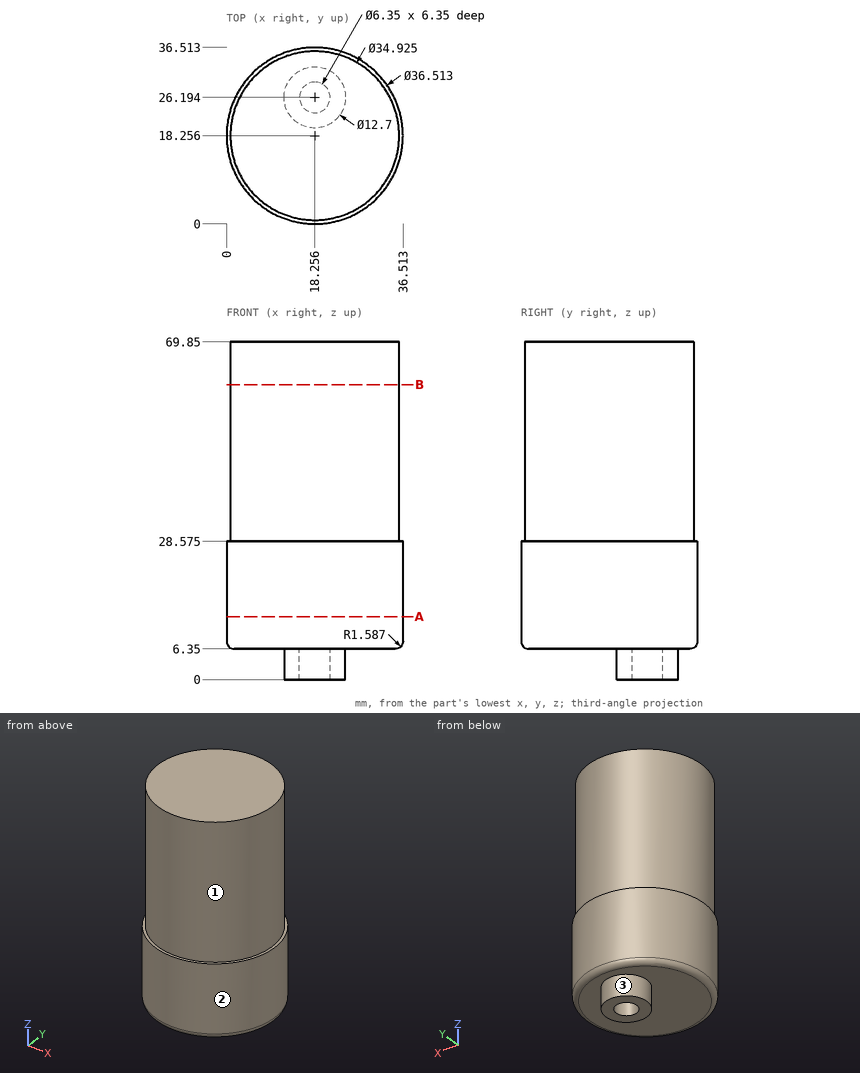
Part print with two shaded views. Sizes in mm from the minimum x, y, z corner. A direction names the side the tool comes from. Coordinates: 2 decimals unless noted, no trailing zeros. Order: outer loops, then holes, each group sorted by start corner. A loop starts at its lowest first (then second) coordinate and runs counter-clockwise, first axis right, second up. Notation, with made-up numbers: (82.25, 67.25) - (114.25, 67.25) arc R29 ccw to (114.25, 94.25) - close; hole circle Ø10 at (69, 55.5). An arc over 180 degrees is marked (long way). Answer in a Markdown table with one row per item.
1. Slice it at A-A, the plane z = 13. List the corners of the cut face in (x, y).
Answer:
| item | result |
|---|---|
| outline | circle Ø36.51 at (18.26, 18.26) |
2. Flat gauge pins, fed straight in: P1, Ø1, axis at x = 24, z = 31.5, coming from the -Y side; P2, Ø6, axis at x = 19, y = 28.5, coming from the -Z side; P3, Ø8, axis at y = 29.5, z = 51.5, coming from the +X side (1 decimal); P4, Ø6, axis at y = 16.5, z = 36, coming from the +X side. Where does each tip first touch, or does it go through?
Answer:
| item | result |
|---|---|
| P1 | y = 1.6 |
| P2 | z = 0 |
| P3 | x = 34.1 |
| P4 | x = 35.72 |
3. Drill centre lines: L1, parallel to Z at x = 2, y = 18.5; L2, parallel to X at y = 26, z = 3.5 (1 decimal); L3, parallel to X at y = 18.5, z = 34 (1 decimal). Where is each one in solid material? Low to high. Write a range as from..to.
Answer:
| item | result |
|---|---|
| L1 | 6.35..69.85 |
| L2 | 11.9..15.1, 21.4..24.6 |
| L3 | 0.8..35.7 |
4. Slice it at B-B, the plane z = 61. List the corners of the cut face in (x, y) (1 decimal).
Answer:
| item | result |
|---|---|
| outline | circle Ø34.9 at (18.3, 18.3) |
5. 3-axis set-ups, long thin cutter, end or side, ignore diameter. For the marked faces 1, 2 and 3: which of +Z, -Z, +X, -X, +Y, -Y reach the whole face in a straight line?
Answer:
| item | result |
|---|---|
| face 1 | +Z |
| face 2 | +Z, -Z |
| face 3 | -Z |
